Input: part model. Units: mm. Frame: model coordinates. Give positions to 0.01 mm unless a question says otherwise; leave off trailing zeros. Loops run counter-clockwise (first coordinate to the right, second up) from the corner with the lowest first, then second, coordinate; pieces in that order, holes last. Notation, with made-up numbers: (39, 39) -> (44, 39) arc R25 ccw to (44, 78) -> close; hole circle Ø5 at (-12.75, 45.25). An arc over 180 degrees is marked (long way). One line per question, with ' | ' between items.
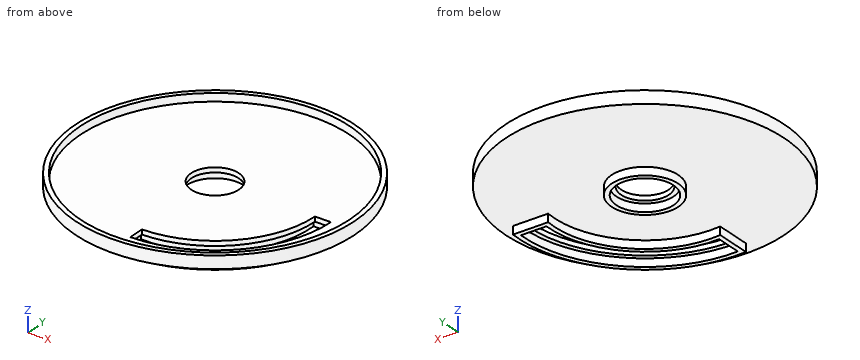
from build123d import *

# Parameters (mm, degrees)
SKETCH_1_R          = 87.6
EXTRUDE_1_DEPTH     = 3
SKETCH_3_R          = 87.6
SKETCH_3_R_2        = 84.6
EXTRUDE_2_DEPTH     = 5
CUT_EXTRUDE_1_DEPTH = 5
EXTRUDE_3_DEPTH     = 5
SKETCH_6_R          = 14.982595121
CUT_EXTRUDE_2_DEPTH = 5
SKETCH_7_R          = 20.982595121
SKETCH_7_R_2        = 17.982595121
EXTRUDE_4_DEPTH     = 5


with BuildPart() as part:
    # 스케치1 → 보스-돌출1 (new body)
    with BuildSketch(Plane.XY):
        Circle(SKETCH_1_R)
    extrude(amount=EXTRUDE_1_DEPTH)

    # 스케치3 → 보스-돌출2 (add)
    with BuildSketch(Plane.XY.offset(3)):
        Circle(SKETCH_3_R)
        Circle(SKETCH_3_R_2, mode=Mode.SUBTRACT)
    extrude(amount=EXTRUDE_2_DEPTH)

    # 스케치4 → 컷-돌출1 (cut)
    with BuildSketch(Plane(origin=(0, 0, 0), x_dir=(-1, 0, 0), z_dir=(0, 0, -1))):
        with BuildLine():
            Line((-63, 0), (-73.1, 0))
            ThreePointArc((-73.1, 0), (-51.689505705, -51.689505705), (0, -73.1))
            Line((0, -73.1), (0, -63))
            ThreePointArc((0, -63), (-44.547727215, -44.547727215), (-63, 0))
        make_face()
    extrude(amount=-CUT_EXTRUDE_1_DEPTH, mode=Mode.SUBTRACT)

    # 스케치5 → 보스-돌출3 (add)
    with BuildSketch(Plane(origin=(0, 0, 0), x_dir=(-1, 0, 0), z_dir=(0, 0, -1))):
        with BuildLine():
            Line((6, -78.872111675), (6, -56.683330883))
            ThreePointArc((6, -56.683330883), (-40.305086528, -40.305086528), (-56.683330883, 6))
            Line((-56.683330883, 6), (-78.872111675, 6))
            ThreePointArc((-78.872111675, 6), (-55.932146392, -55.932146392), (6, -78.872111675))
        make_face()
        with BuildLine():
            Line((-59.924953066, 3), (-76.040844288, 3))
            ThreePointArc((-76.040844288, 3), (-53.810826048, -53.810826048), (3, -76.040844288))
            Line((3, -76.040844288), (3, -59.924953066))
            ThreePointArc((3, -59.924953066), (-42.426406871, -42.426406871), (-59.924953066, 3))
        make_face(mode=Mode.SUBTRACT)
    extrude(amount=EXTRUDE_3_DEPTH)

    # 스케치6 → 컷-돌출2 (cut)
    with BuildSketch(Plane(origin=(0, 0, 0), x_dir=(-1, 0, 0), z_dir=(0, 0, -1))):
        Circle(SKETCH_6_R)
    extrude(amount=-CUT_EXTRUDE_2_DEPTH, mode=Mode.SUBTRACT)

    # 스케치7 → 보스-돌출4 (add)
    with BuildSketch(Plane(origin=(0, 0, 0), x_dir=(-1, 0, 0), z_dir=(0, 0, -1))):
        with Locations(Location((0, 0, 0), (0, 0, 180))):
            Circle(SKETCH_7_R)
        Circle(SKETCH_7_R_2, mode=Mode.SUBTRACT)
    extrude(amount=EXTRUDE_4_DEPTH)


solid = part.part
1. Pin query (flat end, axial travel): P1, Ø6, axis at y = 9, z = -3.5, coming from the -X side; P2, Ø5.5, axis at y = -64, z = -1.5, coming from the +X side; P3, Ø1.5, axis at x = -30, y = 56, coming from the +Z side. Return the tip coordinate at first contact, or that it passes through.
Determined:
P1: stops at x = -20.11 | P2: stops at x = 62.19 | P3: stops at z = 3
2. Section query B-B (x = 6). Count the separate pieces of the cut face and the enclosed holes in it, then the cut area to 3 significant figures.
Determined:
separate pieces: 3 | enclosed holes: 0 | area: 503 mm2
3. Ray query, line 1 along Y through (x, z) = (0, -2.9); line 2 along Y through (x, z) = (0, 5); line 3 along X through (y, z) = (-15.5, -1). Return the intervals inside material, ascending. Write a range as from..to.
Determined:
line 1: y = -79.1..-76.1, -60..-57, -20.98..-17.98, 17.98..20.98 | line 2: y = -87.6..-84.6, 84.6..87.6 | line 3: x = -14.14..-9.12, 9.12..14.14, 54.85..57.96, 74.5..77.57
4. Section query A-A (y = 10). Output: boundary loops of the cut face in (x, z), then the cut area to 3 significant figures.
Determined:
outline: (-87.03, 0) -> (-18.45, 0) -> (-18.45, -5) -> (-14.95, -5) -> (-14.95, 0) -> (-11.16, 0) -> (-11.16, 3) -> (-84.01, 3) -> (-84.01, 8) -> (-87.03, 8) -> close; (11.16, 0) -> (14.95, 0) -> (14.95, -5) -> (18.45, -5) -> (18.45, 0) -> (87.03, 0) -> (87.03, 8) -> (84.01, 8) -> (84.01, 3) -> (11.16, 3) -> close | area: 520 mm2
5. Section query C-C (x = 51.5). Output: boundary loops of the cut face in (y, z), then the cut area to 3 significant figures.
Determined:
outline: (-70.86, 0) -> (-60.04, 0) -> (-60.04, -5) -> (-56.03, -5) -> (-56.03, 0) -> (-51.88, 0) -> (-51.88, 3) -> (-67.12, 3) -> (-67.12, 8) -> (-70.86, 8) -> close; (-36.29, 0) -> (-30.79, 0) -> (-30.79, -5) -> (-24.43, -5) -> (-24.43, 0) -> (70.86, 0) -> (70.86, 8) -> (67.12, 8) -> (67.12, 3) -> (-36.29, 3) -> close | area: 468 mm2
